Verification items for the finished model (mm, model axes). A direction names the side the tool comes from. Coordinates: 2 decimals unless noted, no trailing zeros. Write each loop counter-clockwise with the first axis right and the second up, starting at its lowest first coordinate (ties: lowest second). Pieces come first, ordered by that corner, then holes.
```python
from build123d import *

# Parameters (mm, degrees)
EXTRUDE_1_DEPTH          = 2
SKETCH_1_4_R             = 3
EXTRUDE_2_DEPTH          = 2
CUT_EXTRUDE_1_DEPTH      = 51.040969284
CUT_EXTRUDE_1_DEPTH_BACK = 51.040969284
SKETCH_1_3_R             = 2
FILLET_1_R               = 3
EXTRUDE_START            = -2
SKETCH_2_R               = 2
EXTRUDE_3_DEPTH          = 2
SKETCH_2_3_R             = 1.8
EXTRUDE_4_DEPTH          = 2
EXTRUDE_6_DEPTH          = 2
EXTRUDE_START_2          = -5.5
EXTRUDE_5_DEPTH          = 5.5
FILLET_3_R               = 10


with BuildPart() as part:
    # 草图1 → 凸台-拉伸1 (new body)
    with BuildSketch(Plane(origin=(0, 0, 0), x_dir=(0, 0, -1), z_dir=(1, 0, 0))):
        with BuildLine():
            Line((40.737143614, 0), (0, 0))
            Line((0, 0), (2.48051592, -3.542543867))
            ThreePointArc((2.48051592, -3.542543867), (4.165783411, -4.487079684), (5.367176995, -6))
            Line((5.367176995, -6), (44.201245229, -6))
            ThreePointArc((44.201245229, -6), (40.737143614, -4), (40.737143614, 0))
        make_face()
        with BuildLine():
            Line((2.48051592, -3.542543867), (0, 0))
            Line((0, 0), (-2.681672007, 3.829824531))
            ThreePointArc((-2.681672007, 3.829824531), (-4.811127311, -0.102785303), (-9.234888361, -0.758786959))
            Line((-9.234888361, -0.758786959), (-4.072700434, -8.131155358))
            ThreePointArc((-4.072700434, -8.131155358), (-1.94324513, -4.198545524), (2.48051592, -3.542543867))
        make_face()
        with BuildLine():
            ThreePointArc((48.201245229, -2), (45.23652141, 1.863703305), (40.737143614, 0))
            Line((40.737143614, 0), (44.201245229, 0))
            ThreePointArc((44.201245229, 0), (45.615458792, -0.585786438), (46.201245229, -2))
            ThreePointArc((46.201245229, -2), (45.615458792, -3.414213562), (44.201245229, -4))
            Line((44.201245229, -4), (44.201245229, -6))
            ThreePointArc((44.201245229, -6), (47.029672354, -4.828427125), (48.201245229, -2))
        make_face()
        with BuildLine():
            Line((44.201245229, 0), (40.737143614, 0))
            ThreePointArc((40.737143614, 0), (40.737143614, -4), (44.201245229, -6))
            Line((44.201245229, -6), (44.201245229, -4))
            ThreePointArc((44.201245229, -4), (42.201245229, -2), (44.201245229, 0))
        make_face()
        with BuildLine():
            ThreePointArc((5.367176995, -6), (4.165783411, -4.487079684), (2.48051592, -3.542543867))
            Line((2.48051592, -3.542543867), (4.201245229, -6))
            Line((4.201245229, -6), (5.367176995, -6))
        make_face()
        with BuildLine():
            Line((4.201245229, -6), (2.48051592, -3.542543867))
            ThreePointArc((2.48051592, -3.542543867), (-1.94324513, -4.198545524), (-4.072700434, -8.131155358))
            Line((-4.072700434, -8.131155358), (-2.351971125, -10.588611491))
            Line((-2.351971125, -10.588611491), (-1.532819081, -10.015035054))
            ThreePointArc((-1.532819081, -10.015035054), (-0.796092257, -5.836849613), (3.382093185, -6.573576436))
            Line((3.382093185, -6.573576436), (4.201245229, -6))
        make_face()
        with BuildLine():
            ThreePointArc((-9.234888361, -0.758786959), (-4.811127311, -0.102785303), (-2.681672007, 3.829824531))
            Line((-2.681672007, 3.829824531), (-4.402401316, 6.287280664))
            Line((-4.402401316, 6.287280664), (-6.040705405, 5.140127792))
            ThreePointArc((-6.040705405, 5.140127792), (-5.771575592, 4.594386518), (-5.679009493, 3.992974919))
            ThreePointArc((-5.679009493, 3.992974919), (-7.077597894, 2.085541017), (-9.317313582, 2.845822046))
            Line((-9.317313582, 2.845822046), (-10.95561767, 1.698669174))
            Line((-10.95561767, 1.698669174), (-9.234888361, -0.758786959))
        make_face()
        with BuildLine():
            Line((-4.402401316, 6.287280664), (-2.681672007, 3.829824531))
            ThreePointArc((-2.681672007, 3.829824531), (-2.679675166, 3.911388863), (-2.679009493, 3.992974919))
            ThreePointArc((-2.679009493, 3.992974919), (-10.613341245, 8.041394014), (-9.234888361, -0.758786959))
            Line((-9.234888361, -0.758786959), (-10.95561767, 1.698669174))
            Line((-10.95561767, 1.698669174), (-9.317313582, 2.845822046))
            ThreePointArc((-9.317313582, 2.845822046), (-8.826162366, 5.631279008), (-6.040705405, 5.140127792))
            Line((-6.040705405, 5.140127792), (-4.402401316, 6.287280664))
        make_face()
        with BuildLine():
            ThreePointArc((46.201245229, -2), (45.615458792, -0.585786438), (44.201245229, 0))
            Line((44.201245229, 0), (44.201245229, -4))
            ThreePointArc((44.201245229, -4), (45.615458792, -3.414213562), (46.201245229, -2))
        make_face()
        with BuildLine():
            Line((44.201245229, -4), (44.201245229, 0))
            ThreePointArc((44.201245229, 0), (42.201245229, -2), (44.201245229, -4))
        make_face()
        with BuildLine():
            Line((5.367176995, -6), (4.201245229, -6))
            Line((4.201245229, -6), (3.382093185, -6.573576436))
            ThreePointArc((3.382093185, -6.573576436), (3.785787904, -7.392188347), (3.924637052, -8.294305745))
            ThreePointArc((3.924637052, -8.294305745), (1.826754451, -11.155456598), (-1.532819081, -10.015035054))
            Line((-1.532819081, -10.015035054), (-2.351971125, -10.588611491))
            Line((-2.351971125, -10.588611491), (-4.072700434, -8.131155358))
            ThreePointArc((-4.072700434, -8.131155358), (0.843050996, -13.293640073), (5.924637052, -8.294305745))
            ThreePointArc((5.924637052, -8.294305745), (5.783273678, -7.113776143), (5.367176995, -6))
        make_face()
        with BuildLine():
            ThreePointArc((3.924637052, -8.294305745), (3.785787904, -7.392188347), (3.382093185, -6.573576436))
            Line((3.382093185, -6.573576436), (2.562941141, -7.147152873))
            ThreePointArc((2.562941141, -7.147152873), (2.832070954, -7.692894146), (2.924637052, -8.294305745))
            ThreePointArc((2.924637052, -8.294305745), (1.526048651, -10.201739647), (-0.713667036, -9.441458618))
            Line((-0.713667036, -9.441458618), (-1.532819081, -10.015035054))
            ThreePointArc((-1.532819081, -10.015035054), (1.826754451, -11.155456598), (3.924637052, -8.294305745))
        make_face()
        with BuildLine():
            Line((2.562941141, -7.147152873), (3.382093185, -6.573576436))
            ThreePointArc((3.382093185, -6.573576436), (-0.796092257, -5.836849613), (-1.532819081, -10.015035054))
            Line((-1.532819081, -10.015035054), (-0.713667036, -9.441458618))
            ThreePointArc((-0.713667036, -9.441458618), (-0.222515821, -6.656001657), (2.562941141, -7.147152873))
        make_face()
        with BuildLine():
            ThreePointArc((-5.679009493, 3.992974919), (-5.771575592, 4.594386518), (-6.040705405, 5.140127792))
            Line((-6.040705405, 5.140127792), (-9.317313582, 2.845822046))
            ThreePointArc((-9.317313582, 2.845822046), (-7.077597894, 2.085541017), (-5.679009493, 3.992974919))
        make_face()
        with BuildLine():
            Line((-9.317313582, 2.845822046), (-6.040705405, 5.140127792))
            ThreePointArc((-6.040705405, 5.140127792), (-8.826162366, 5.631279008), (-9.317313582, 2.845822046))
        make_face()
        with BuildLine():
            ThreePointArc((2.924637052, -8.294305745), (2.832070954, -7.692894146), (2.562941141, -7.147152873))
            Line((2.562941141, -7.147152873), (-0.713667036, -9.441458618))
            ThreePointArc((-0.713667036, -9.441458618), (1.526048651, -10.201739647), (2.924637052, -8.294305745))
        make_face()
        with BuildLine():
            Line((-0.713667036, -9.441458618), (2.562941141, -7.147152873))
            ThreePointArc((2.562941141, -7.147152873), (-0.222515821, -6.656001657), (-0.713667036, -9.441458618))
        make_face()
    extrude(amount=EXTRUDE_1_DEPTH)

    # 草图1<4> → 凸台-拉伸2 (add)
    with BuildSketch(Plane(origin=(0, 0, 0), x_dir=(0, 0, -1), z_dir=(1, 0, 0))):
        with Locations((0.924637052, -8.294305745)):
            Circle(SKETCH_1_4_R)
    extrude(amount=-EXTRUDE_2_DEPTH)

    # 草图1<3> → 切除-拉伸1 (cut, two sides: drawn at the far end of the back side and taken through both)
    with BuildSketch(Plane(origin=(0, 0, 0), x_dir=(0, 0, -1), z_dir=(1, 0, 0)).offset(-CUT_EXTRUDE_1_DEPTH_BACK)):
        with Locations((-7.679009493, 3.992974919)):
            Circle(SKETCH_1_3_R)
        with Locations((44.201245229, -2)):
            Circle(SKETCH_1_3_R)
        with Locations((0.924637052, -8.294305745)):
            Circle(SKETCH_1_3_R)
    extrude(amount=CUT_EXTRUDE_1_DEPTH + CUT_EXTRUDE_1_DEPTH_BACK, mode=Mode.SUBTRACT)

    # 圆角1
    fillet_1_edges = [part.edges().sort_by_distance(p)[0] for p in [
        (1, -6, -5.367176995),
        (1, 0, 0),
        (1, 0, -40.737143614),
        (1, -0.758786959, 9.234888361),
        (1, -8.131155358, 4.072700434),
    ]]
    fillet(fillet_1_edges, radius=FILLET_1_R)

    # 草图2 → 凸台-拉伸3 (add)
    with BuildSketch(Plane(origin=(2, 0, 0), x_dir=(0, 0, -1), z_dir=(1, 0, 0)).offset(EXTRUDE_START)):
        with Locations((-7.679009493, 3.992974919)):
            Circle(SKETCH_2_R)
    extrude(amount=EXTRUDE_3_DEPTH)

    # 草图2<3> → 凸台-拉伸4 (add)
    with BuildSketch(Plane(origin=(2, 0, 0), x_dir=(0, 0, -1), z_dir=(1, 0, 0))):
        with Locations((-7.679009493, 3.992974919)):
            Circle(SKETCH_2_3_R)
    extrude(amount=EXTRUDE_4_DEPTH)

    # 草图4 → 凸台-拉伸6 (add)
    with BuildSketch(Plane(origin=(2, 0, 0), x_dir=(0, 0, -1), z_dir=(1, 0, 0))):
        Polygon((-5.244772745, 8.360410259), (9.755227255, 0), (-5.244772745, 0), align=None)
    extrude(amount=-EXTRUDE_6_DEPTH)

    # 草图3 → 凸台-拉伸5 (add)
    with BuildSketch(Plane(origin=(2, 0, 0), x_dir=(0, 0, -1), z_dir=(1, 0, 0)).offset(EXTRUDE_START_2)):
        with BuildLine():
            Line((-12.894335644, 6.959517206), (-12.261585188, 5.992974919))
            ThreePointArc((-12.261585188, 5.992974919), (-10.417622281, 8.176275052), (-7.679009493, 8.992974919))
            Line((-7.679009493, 8.992974919), (-8.311759949, 9.959517206))
            ThreePointArc((-8.311759949, 9.959517206), (-10.965344838, 9.012935078), (-12.894335644, 6.959517206))
        make_face()
    extrude(amount=EXTRUDE_5_DEPTH)

    # 圆角3
    fillet_3_edges = [part.edges().sort_by_distance(p)[0] for p in [
        (1, 0, -9.755227255),
    ]]
    fillet(fillet_3_edges, radius=FILLET_3_R)

    # 镜向1: part across plane


with BuildPart() as part_1:
    add(part.part)
    add(part.part.mirror(Plane.ZY.offset(3.5)))


solid = part_1.part
```
1. Gauge pin test, flat ends, axial feed: P1, Ø1.5, axis at x = 0, z = -36, coming from the -Y side; P2, Ø3, axis at y = -5, z = -7, coming from the -X side; P3, Ø7, axis at y = -4.5, z = -27.5, coming from the +X side; P4, Ø5, axis at x = 1, y = -0.5, coming from the -Z side. Record the tip position at first contact, or that the pin passes through.
2. Sectioned sample at C-C, the plane y = 5. Record the boundary of the cut face in (x, z), and give its area (3 significant figures).
3. Material ranges on L1, parallel to Z at x = 1.05, y = -2; L2, parallel to X at y = -5.75, z = -23; L3, parallel to Y at x = -7.25, z = -43, recorded low to high.
4. Tool access check on faces 1 (the cylindrical face through (1.014, -8.075, 4.225)), 2 (the cylindrical face through (-6.01, -5.32, -0.53)), 3 (the cylindrical face through (-9.99, 5.78, 7.91)), 4 (the cylindrical face through (-6.97, -6.31, -0.66)), 5 (the cylindrical face through (-7.99, 0.33, -9.8)). Record the directions out of +Z, -Z, +X, -X, +Y, -Y that give a thin tool (end or side, any length) a straight path to the whole face; none if there is none.
5. Sectioned sample at A-A, the plane z = 7. Record the boundary of the cut face in (x, y).
6. Sectioned sample at B-B, the plane x = -0.75. Record the boundary of the cut face in (y, z).
7. Draft check along X on faces 6 (the cylindrical face through (0.99, 0.33, -9.8)), 7 (the flat face through (2, -2, -13)), 8 (the flat face through (0, -1, -11)). Enter one of: pulls with the +X half, pulls with the -X half, needs draft (parallel to the pull), parting line crosses it, or undercut.
Outcome:
1. P1: stops at y = -6
1. P2: stops at x = -9
1. P3: stops at x = 2
1. P4: stops at z = -48.2
2. outline: (-11, 6.19) - (-9, 6.19) - (-9, -0.78) - (-7, -0.78) - (-7, 12.58) - (-9, 12.58) - (-9, 9.17) - (-11, 9.17) - close; (0, -0.78) - (2, -0.78) - (2, 6.19) - (4, 6.19) - (4, 9.17) - (2, 9.17) - (2, 12.58) - (0, 12.58) - close
2. area: 65.4 mm2
3. L1: z = -48.2 to -46.2, -42.2 to 8.37
3. L2: x = -9 to -7, 0 to 2
3. L3: y = -6 to -3.6, -0.4 to 1.82
4. face 1: +Z, +X, -X, -Y
4. face 2: none
4. face 3: -X
4. face 4: +X, -X
4. face 5: +X, -X, +Y
5. outline: (-11, 2.33) - (-9, 2.33) - (-9, -3.95) - (-7, -3.95) - (-7, 8.95) - (-9, 8.95) - (-9, 5.66) - (-11, 5.66) - close; (0, -3.95) - (2, -3.95) - (2, 2.33) - (4, 2.33) - (4, 5.66) - (2, 5.66) - (2, 8.95) - (0, 8.95) - close
6. outline: circle Ø6 at (-8.29, -0.92); (5.99, 12.26) arc R5 cw to (8.99, 7.68) - (9.96, 8.31) arc R6 ccw to (6.96, 12.89) - close; hole circle Ø4 at (-8.29, -0.92)
7. face 6: needs draft
7. face 7: pulls with the +X half
7. face 8: undercut
